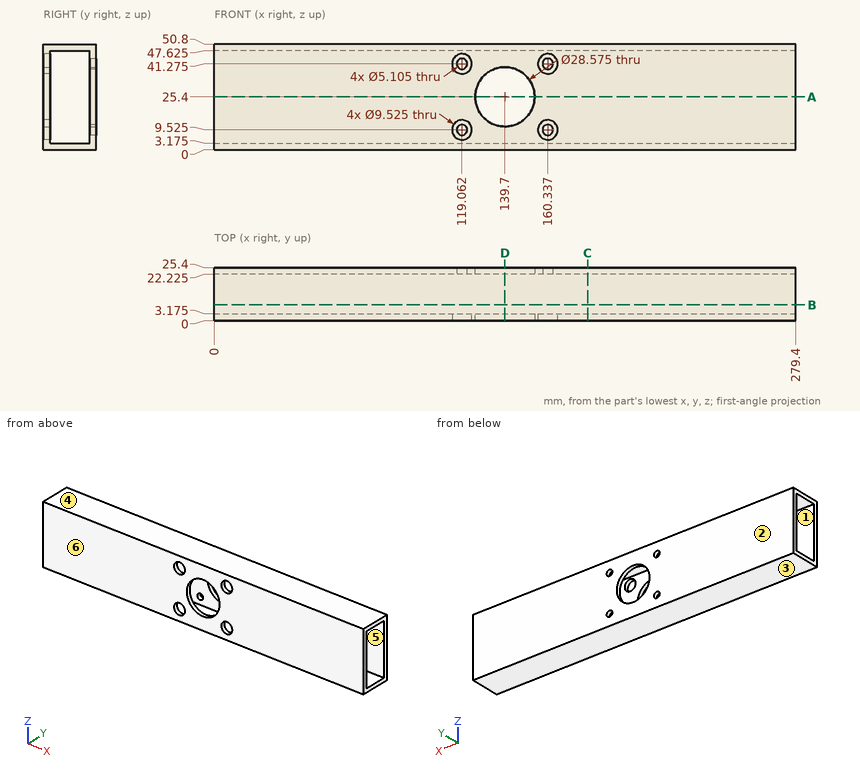
Could you check a few things on this drawing? It's one solid part, dimensions in mm from its lowest x, y, z. A direction names the side the tool comes from. Round coordinates to 2 decimals unless told otherwise and drop trailing zeros. Loops run counter-clockwise (first coordinate to the right, second up) from the corner with the lowest first, then second, coordinate; pieces in that order, holes last. Notation, with made-up numbers: M -20,62 L -7,62 A17 cw -7,90 Z; hole C 75,40.25 d5. An arc over 180 degrees is marked long. Write item = value, one per line. Start each with the question number.
(1) Suppose I cut it at A-A on z = 25.4. Write out the boundary of the cut face in (x, y) (1 decimal).
(2) Suppose I cut it at D-D on x = 139.7. Write out the boundary of the cut face in (y, z) (1 decimal).
(3) If we mould it in two halves opening along Z, with no side actions, what happens to the marked faces 3, 4, 5 and 6? For each: released by +Z, released by -Z, zero draft, split by the parting line, or undercut.
(4) Suppose I cut it at C-C on x = 179.5. Write out the boundary of the cut face in (y, z) (1 decimal).
(5) Suppose I cut it at B-B on y = 7.5. Write out the boundary of the cut face in (x, z) (1 decimal).
(6) I'm going to push flat-ended pins straight in: P1, Ø1, axis at x = 123.5, z = 17, coming from the -Y side; P2, Ø4, axis at x = 119.06, z = 9.52, coming from the -Y side; P3, Ø8, axis at x = 119.06, z = 41.28, coming from the -Y side (1 decimal). Where does each tip first touch, or does it pass through?
(7) I need wall thicknesses on line 1 along Z through (x, y) = (171, 16.5) (1 decimal); line 2 along Y through (x, z) = (101, 7) (1 decimal). Which ranges of each line are inside material? Lowest first, please.
(8) Which directions (+Z, -Z, +X, -X, +Y, -Y) give clear straight access to the entire face, cutting with the end or side of a thin tool? Please do the marked faces 1 and 2.
Answer block:
q1.outline = M 0,0 L 125.4,0 L 125.4,3.2 L 0,3.2 Z; M 0,22.2 L 125.4,22.2 L 125.4,25.4 L 0,25.4 Z; M 154,0 L 279.4,0 L 279.4,3.2 L 154,3.2 Z; M 154,22.2 L 279.4,22.2 L 279.4,25.4 L 154,25.4 Z
q2.outline = M 0,0 L 25.4,0 L 25.4,11.1 L 22.2,11.1 L 22.2,3.2 L 3.2,3.2 L 3.2,11.1 L 0,11.1 Z; M 0,39.7 L 3.2,39.7 L 3.2,47.6 L 22.2,47.6 L 22.2,39.7 L 25.4,39.7 L 25.4,50.8 L 0,50.8 Z
q3.face_3 = released by -Z
q3.face_4 = released by +Z
q3.face_5 = undercut
q3.face_6 = zero draft
q4.outline = M 0,0 L 25.4,0 L 25.4,50.8 L 0,50.8 Z; hole M 3.2,3.2 L 22.2,3.2 L 22.2,47.6 L 3.2,47.6 Z
q5.outline = M 0,0 L 279.4,0 L 279.4,3.2 L 0,3.2 Z; M 0,47.6 L 279.4,47.6 L 279.4,50.8 L 0,50.8 Z
q6.P1 = 0
q6.P2 = through
q6.P3 = 22.2
q7.line_1 = 0 to 3.2, 47.6 to 50.8
q7.line_2 = 0 to 3.2, 22.2 to 25.4
q8.face_1 = +X, -X
q8.face_2 = +Z, -Z, +X, -X, +Y
